Build history of the part. All positions in model axes, mm. A direction names the side the tool comes from. Round coordinates to 2 decimals unless told otherwise and drop trailing zeros. Order: outer loops, then holes, each group sorted by start corner. A loop starts at its lowest first (then second) coordinate and runs counter-clockwise, first axis right, second up. Notation, with made-up numbers: (37, 48) -> (52, 48) arc R22 ccw to (52, 65) -> close; hole circle Ø11 at (20.5, 32.25). An arc over 180 degrees is marked (long way). Use a Markdown table: item, result. Add a question column.
Item 1: Slice it at A-A, the plane z = 20.5. Give the cut face in (x, y).
Item 2: Slice it at C-C, the plane z = -16. Give the cut face in (x, y).
Item 3: 3-axis set-ups, long thin cutter, end or side, ignore diameter. For faces 1 (the face through (39, -13, 22)), 2 (the face through (39.57, -26.4, 21.81)), 3 (the face through (40, -13, 26.25)), 4 (the face through (3.43, -0.6, 26.37)): which of +Z, -Z, +X, -X, +Y, -Y reach the whole face in a straight line?
Item 4: Pin check, flat tips, straight feed: pin 1 (1 mm diameter, centred on x = 38, y = -23, fed in from -Z); pin 2 (12 mm diameter, centred on x = 8.5, y = -4.5, fed in from +Z); pin 3 (10 mm diameter, centred on x = 37, y = -3, fed in from +Z). Stop position of each tip, or through.
Item 5: Two-plate mould, pull along X, no slides. Class faces 5 (the face through (42.43, -13.69, 25.65)), 6 (the face through (13.4, -27, -0.5)), 7 (the face through (3.43, -26.4, 26.37)): released by +X, released by -X, zero draft, split by the parting line, or undercut.
Item 6: Probe L1, parallel to X at y = -15, z = 19; L2, parallel to X at y = -14.75, z = -24.5; L3, parallel to X at y = -24, z = 4.5. List the from-to ranges inside material, lowest first.
Item 7: Slice it at B-B, the plane y = -12.25. Give the cut face in (x, z).
from build123d import *

# Parameters (mm, degrees)
F1_W     = 4
F1_H     = 42
F1_H_2   = 8.75
F2_DEPTH = 27
F3_R     = 1.99999


# Not quite as in the source:
# - a fillet or chamfer is up to 0.001 mm smaller than in the source, because OpenCascade refuses the exact size


with BuildPart() as f2:
    # F1 (on Front) → F2 (new body)
    with BuildSketch(Plane.XZ):
        with BuildLine():
            Line((4, 35), (0, 35))
            Line((0, 35), (0, 17.5))
            ThreePointArc((0, 17.5), (1.0244047706, 24.0574385243), (4, 29.9899959968))
            Line((4, 29.9899959968), (4, 35))
        make_face()
        with BuildLine():
            ThreePointArc((4, 5.0100040032), (1.0244047706, 10.9425614757), (0, 17.5))
            Line((0, 17.5), (0, 0))
            Line((0, 0), (4, 0))
            Line((4, 0), (4, 5.0100040032))
        make_face()
        with BuildLine():
            Line((4, 17.5), (0, 17.5))
            ThreePointArc((0, 17.5), (1.0244047706, 10.9425614757), (4, 5.0100040032))
            Line((4, 5.0100040032), (4, 17.5))
        make_face()
        with BuildLine():
            ThreePointArc((4, 29.9899959968), (1.0244047706, 24.0574385243), (0, 17.5))
            Line((0, 17.5), (4, 17.5))
            Line((4, 17.5), (4, 29.9899959968))
        make_face()
        with Locations((2, -21)):
            Rectangle(F1_W, F1_H)
        with BuildLine():
            ThreePointArc((9.0100040032, 0), (6.2972042045, 2.2972042045), (4, 5.0100040032))
            Line((4, 5.0100040032), (4, 0))
            Line((4, 0), (9.0100040032, 0))
        make_face()
        with BuildLine():
            Line((4, 17.5), (4, 5.0100040032))
            ThreePointArc((4, 5.0100040032), (6.2972042045, 2.2972042045), (9.0100040032, 0))
            Line((9.0100040032, 0), (21.5, 0))
            ThreePointArc((21.5, 0), (9.1256313292, 5.1256313292), (4, 17.5))
        make_face()
        with BuildLine():
            Line((21.5, 0), (9.0100040032, 0))
            ThreePointArc((9.0100040032, 0), (21.5, -4), (33.9899959968, 0))
            Line((33.9899959968, 0), (21.5, 0))
        make_face()
        with BuildLine():
            ThreePointArc((39, 17.5), (33.8743686708, 5.1256313292), (21.5, 0))
            Line((21.5, 0), (33.9899959968, 0))
            ThreePointArc((33.9899959968, 0), (40.6152414833, 7.6583770122), (43, 17.5))
            Line((43, 17.5), (39, 17.5))
        make_face()
        with Locations((41, 21.875)):
            Rectangle(F1_W, F1_H_2)
    extrude(amount=F2_DEPTH)

    # F3 (radius 2 in the source; OpenCascade refuses exactly that, so slightly less here)
    f3_edges = [f2.edges().sort_by_distance(p)[0] for p in [
        (4, -27, -21),
        (4, -27, 26.25),
        (4, 0, -21),
        (4, -13.5, -42),
        (4, 0, 26.25),
        (43, -13.5, 26.25),
        (4, -13.5, 35),
    ]]
    fillet(f3_edges, radius=F3_R)


solid = f2.part
Check sheet entries:
| question | item | result |
|---|---|---|
| 1 | outline | (0, -27) -> (2, -27) arc R2 ccw to (4, -25) -> (4, -2) arc R2 ccw to (2, 0) -> (0, 0) -> close; (39, -25) arc R2 ccw to (41, -27) -> (43, -27) -> (43, 0) -> (41, 0) arc R2 ccw to (39, -2) -> close |
| 2 | outline | (0, -27) -> (2, -27) arc R2 ccw to (4, -25) -> (4, -2) arc R2 ccw to (2, 0) -> (0, 0) -> close |
| 3 | face 1 | +Z, +Y, -Y |
| 3 | face 2 | +Z, -Y |
| 3 | face 3 | +Z, +X, +Y, -Y |
| 3 | face 4 | +Z, +Y |
| 4 | pin 1 | z = 3.14 |
| 4 | pin 2 | z = 34.94 |
| 4 | pin 3 | z = 26.25 |
| 5 | face 5 | released by +X |
| 5 | face 6 | zero draft |
| 5 | face 7 | undercut |
| 6 | L1 | 0 to 4, 39 to 43 |
| 6 | L2 | 0 to 4 |
| 6 | L3 | 0 to 9.78, 33.22 to 38.62 |
| 7 | outline | (0, -42) -> (2, -42) arc R2 ccw to (4, -40) -> (4, 0) -> (9.01, 0) arc R21.5 ccw to (43, 17.5) -> (43, 24.25) arc R2 ccw to (41, 26.25) -> (39, 26.25) -> (39, 17.5) arc R17.5 cw to (4, 17.5) -> (4, 33) arc R2 ccw to (2, 35) -> (0, 35) -> close |
